Autodesk Inventor part; units mm, degrees
ref_plane "Plan de construction1" through (30, 0, 0) normal (1, 0, 0) x (0, 1, 0)
ref_plane "Work Plane2" through (0, 0, 30) normal (0, 0, 1) x (1, 0, 0)
ref_plane "XZ Plane" through (0, 0, 0) normal (0, 1, 0) x (-1, 0, 0)
sketch "Esquisse1" plane through (0, 0, 0) normal (0, 1, 0) x (-1, 0, 0)
  circle A0 centre (0, 0) radius 27
  circle A1 centre (0, 0) radius 30
  dimension "d0" = 60
  dimension "d1" = 54
extrude "Extrusion1" add sketch "Esquisse1" along normal blind 150
ref_plane "Plan de construction1" through (30, 0, 0) normal (1, 0, 0) x (0, 1, 0)
sketch "Esquisse2" plane through (30, 0, 0) normal (1, 0, 0) x (0, 1, 0)
  line L0 (56, 6.5) -> (5, 6.5)
  line L1 (5, 6.5) -> (5, -6.5)
  line L2 (5, -6.5) -> (56, -6.5)
  line L3 (56, -6.5) -> (56, 6.5)
  line L4 (0, -27) -> (0, 27)
  line L5 (-11.2, 0) -> (67.2, 0)
  point P0 (0, 0)
  dimension "d5" = 5
  dimension "d6" = 51
  dimension "d7" = 13
  dimension "d8" = 6.5
extrude "Extrusion2" cut sketch "Esquisse2" against normal blind 10
sketch "Esquisse3" plane through (0, 0, 0) normal (0, -1, 0) x (1, 0, 0)
  circle A0 centre (0, 0) radius 27
  arc A1 (0, 27) -> (0, -27) centre (0, 0) ccw
  circle A2 centre (0, 0) radius 30
  arc A3 (0, 30) -> (0, -30) centre (0, 0) ccw
  line L0 (0, 30) -> (0, 27)
  line L1 (0, -30) -> (0, -27)
extrude "Extrusion3" cut sketch "Esquisse3" against normal blind 26 contours A0 L1 A2 L0 picked at (-4.547, -28.4479)
ref_plane "Work Plane2" through (0, 0, 30) normal (0, 0, 1) x (1, 0, 0)
sketch "Sketch4" plane through (0, 0, 30) normal (0, 0, 1) x (1, 0, 0)
  circle A0 centre (-3.6258, 29.618) radius 1.5
  point P0 (0, 0)
extrude "Extrusion4" cut sketch "Sketch4" against normal up to next
properties part number "cylindre-lanceur"
Read the model definition and answer for the solid it produces. Units are mm, in the model's axes. A direction names the side the tool comes from. Round coordinates to 2 decimals unless told otherwise and drop trailing zeros. Order: outer loops, then holes, each group sorted by start corner. A loop starts at its lowest first (then second) coordinate and runs counter-clockwise, first axis right, second up. Notation, with made-up numbers: (-16.5, 41.5) - (40.5, 41.5) arc R26 ccw to (40.5, 77.5) - close; hole circle Ø4 at (80.5, -10.5). An arc over 180 degrees is marked (long way). Use one line per item in the form item = value. Start each with the question number.
(1) Flat-ended cylindrical pins translate along their axes: pin 1 Ø12 at (y, z) = (82, -8) entering from +X; pin 2 Ø6 at (y, z) = (103, 1.5) entering from -X; pin 3 Ø2.5 at (y, z) = (16.5, 28.5) entering from -X; pin 4 Ø5 at (x, y) = (-3.63, 29.62) entering from +Z. Find the tip coordinate at first contact, or state that the pin passes through.
(2) For faces 1 (the face through (-3.951, 28.154, 28.241)), 2 (the face through (28, 56, 0)), 3 (the face through (-27.3, 26, 0.1)), determine the directions among +Z, -Z, +X, -X, +Y, -Y from which every point of the face is accessible in a straight line to the end or side of a thin tool.
(3) Determine the mould class of faces 4 (the face through (0, 13, 29)), 5 (the face through (28, 30, -6.5)), 6 (the face through (29.97, 90.62, -1.32)) for opening direction Z: +Z half, -Z half, draft (parallel to the pull), parting line (faces both ways), or undercut.
(4) The part is cut by section B-B (y = 13). Give the vertices of the cut face in (x, z).
(5) The part is cut by section C-C (x = -7). Give the vertices of the cut face in (y, z), then the cut area to 3 significant figures.
(6) The part is cut by section A-A (z = 0). Give the vertices of the cut face in (x, y), then the cut area to 3 significant figures.
(7) The part is cut by section D-D (y = 116). Give the vertices of the cut face in (x, z).
(8) Find the intervals of material crossed by line 1 along Z through (x, y) = (0, 98); line 2 along Z through (x, y) = (-8, 131), in increasing order. Write a range as from..to.
Checked values:
q1.pin_1 = 29.93
q1.pin_2 = -30
q1.pin_3 = 0
q1.pin_4 = 29.98
q2.face_1 = +Z
q2.face_2 = +X
q2.face_3 = +Z, -Z, -X, -Y
q3.face_4 = draft
q3.face_5 = undercut
q3.face_6 = parting line
q4.outline = (0, -30) arc R30 ccw to (29.29, -6.5) - (26.21, -6.5) arc R27 cw to (0, -27) - close; (0, 27) arc R27 cw to (26.21, 6.5) - (29.29, 6.5) arc R30 ccw to (0, 30) - close
q5.outline = (26, -29.17) - (150, -29.17) - (150, -26.08) - (26, -26.08) - close; (26, 26.08) - (150, 26.08) - (150, 29.17) - (26, 29.17) - close
q5.area = 768 mm^2
q6.outline = (-30, 26) - (-27, 26) - (-27, 150) - (-30, 150) - close; (27, 0) - (30, 0) - (30, 5) - (27, 5) - close; (27, 56) - (30, 56) - (30, 150) - (27, 150) - close
q6.area = 669 mm^2
q7.outline = circle Ø60 at (0, 0); hole circle Ø54 at (0, 0)
q8.line_1 = -30..-27, 27..30
q8.line_2 = -28.91..-25.79, 25.79..28.91
